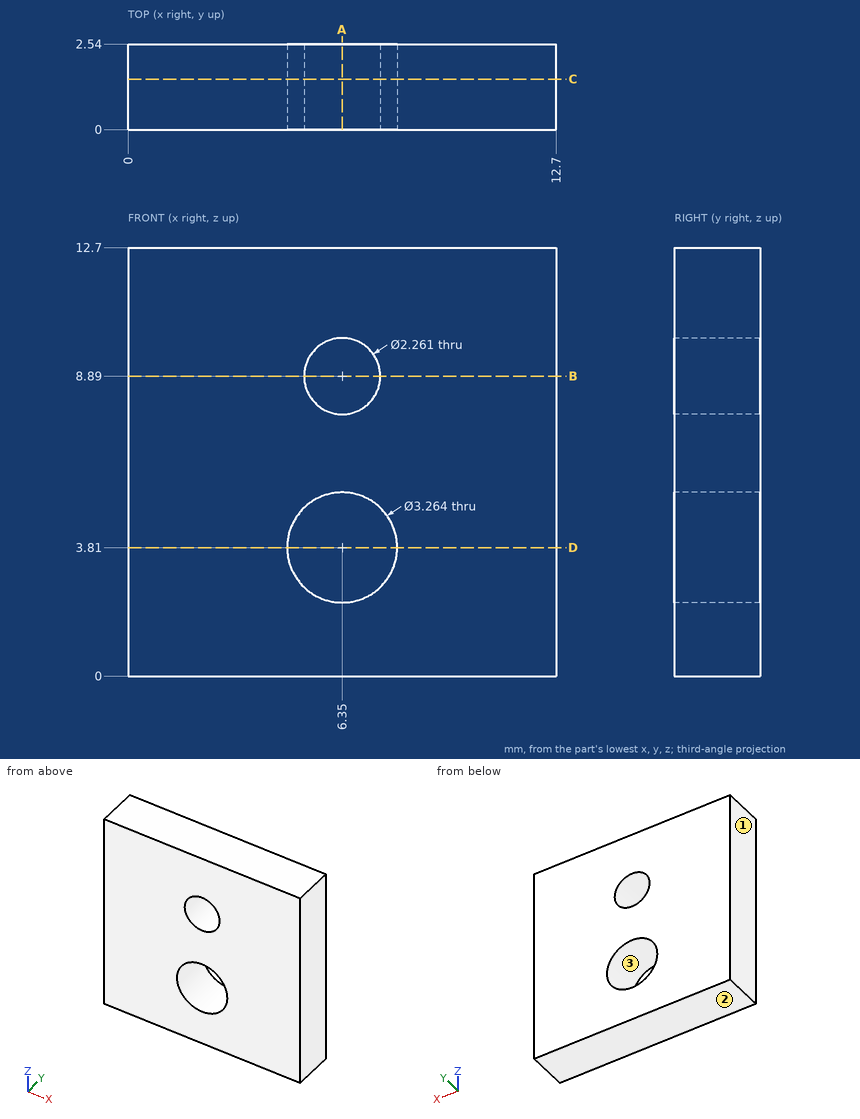
Could you check a few things on this drawing? It's one solid part, dimensions in mm from its lowest x, y, z. Give positions to 0.01 mm unless a question says otherwise; leave off trailing zeros. Write each loop counter-clockwise with the first axis right and the second up, starting at its lowest first coordinate (ties: lowest second). Pieces come first, ordered by that corner, then holes. Notation, with made-up numbers: M 1.25,85.5 L 33.25,85.5 A21 ccw 33.25,97.5 Z; hole C 45,50.5 d1. An arc over 180 degrees is marked long. Put each result on its own line as item: value. Start each with the question number.
Item 1: Thinking about a two-plate mould opening in Z: for the marked faces 1, 2 and 3, which applies, +Z half, -Z half, draft (parallel to the pull), parting line (faces both ways), or undercut?
Item 2: If we section it at A-A, the plane x = 6.35: Write out the boundary of the cut face in (y, z), then the cut area to 3 significant figures.
Item 3: If we section it at D-D, the plane z = 3.81: Write out the boundary of the cut face in (x, y).
Item 4: I need wall thicknesses on L1, parallel to X at y = 1.85, z = 8.89; L2, parallel to X at y = 1.95, z = 3.81; L3, parallel to Z at x = 6.5, y = 1.5 (1 decimal). Which ranges of each line are inside material? Lowest first, please. Write a range as from..to.
Item 5: If we section it at C-C, the plane y = 1.5: Write out the boundary of the cut face in (x, z).
Item 6: If we section it at B-B, the plane z = 8.89: Write out the boundary of the cut face in (x, y).
Values:
1. face 1: draft
1. face 2: -Z half
1. face 3: undercut
2. outline: M 0,0 L 2.54,0 L 2.54,2.18 L 0,2.18 Z; M 0,5.44 L 2.54,5.44 L 2.54,7.76 L 0,7.76 Z; M 0,10.02 L 2.54,10.02 L 2.54,12.7 L 0,12.7 Z
2. area: 18.2 mm²
3. outline: M 0,0 L 4.72,0 L 4.72,2.54 L 0,2.54 Z; M 7.98,0 L 12.7,0 L 12.7,2.54 L 7.98,2.54 Z
4. L1: 0..5.22, 7.48..12.7
4. L2: 0..4.72, 7.98..12.7
4. L3: 0..2.2, 5.4..7.8, 10..12.7
5. outline: M 0,0 L 12.7,0 L 12.7,12.7 L 0,12.7 Z; hole C 6.35,3.81 d3.26; hole C 6.35,8.89 d2.26
6. outline: M 0,0 L 5.22,0 L 5.22,2.54 L 0,2.54 Z; M 7.48,0 L 12.7,0 L 12.7,2.54 L 7.48,2.54 Z
